Autodesk Inventor part; units mm, degrees
ref_plane "YZ Plane" through (0, 0, 0) normal (1, 0, 0) x (0, 1, 0)
ref_plane "XZ Plane" through (0, 0, 0) normal (0, 1, 0) x (-1, 0, 0)
ref_plane "XY Plane" through (0, 0, 0) normal (0, 0, 1) x (1, 0, 0)
sketch "スケッチ1" plane through (0, 0, 0) normal (1, 0, 0) x (0, 1, 0)
  line L0 (13.5, 13.5) -> (-13.5, 13.5)
  line L1 (-13.5, 13.5) -> (-13.5, -13.5)
  line L2 (-13.5, -13.5) -> (13.5, -13.5)
  line L3 (13.5, -13.5) -> (13.5, 13.5)
  circle A0 centre (0, 0) radius 6.5
  circle A1 centre (10.5, 10.5) radius 1.5
  circle A2 centre (10.5, -10.5) radius 1.5
  circle A3 centre (-10.5, -10.5) radius 1.5
  circle A4 centre (-10.5, 10.5) radius 1.5
  dimension "d0" = 27
  dimension "d1" = 27
  dimension "d2" = 13.5
  dimension "d3" = 13.5
  dimension "d4" = 13.5
  dimension "d5" = 13.5
  dimension "d6" = 13
  dimension "d7" = 3
  dimension "d8" = 3
  dimension "d9" = 3
  dimension "d10" = 3
  dimension "d11" = 3
  dimension "d12" = 3
  dimension "d13" = 3
  dimension "d14" = 3
  dimension "d15" = 3
  dimension "d16" = 3
  dimension "d17" = 3
  dimension "d18" = 3
extrude "押し出し1" add sketch "スケッチ1" along normal blind 2
extrude "押し出し2" add sketch "スケッチ1" along normal blind 25 contours A0
fillet "フィレット1" radius 6 1 edges at (25, -6.5, 0)
sketch "スケッチ2" plane through (2, 0, 0) normal (1, 0, 0) x (0, 0, -1)
  circle A0 centre (0, 10) radius 1.5
  circle A1 centre (-10, -6.5) radius 1.5
  circle A2 centre (10, -6.5) radius 1.3994
  line L0 (0, 10) -> (10, -6.5)
  line L1 (10, -6.5) -> (-10, -6.5)
  line L2 (0, 10) -> (-10, -6.5)
  line L3 (13.5, 13.5) -> (-13.5, 13.5)
  line L4 (13.5, -13.5) -> (13.5, 13.5)
  line L5 (-13.5, 13.5) -> (-13.5, -13.5)
  line L6 (-13.5, -13.5) -> (13.5, -13.5)
  point P0 (0, 0)
  dimension "d25" = 3.5
  dimension "d26" = 3.5
  dimension "d27" = 3.5
  dimension "d28" = 2.7988
  dimension "d29" = 7
  dimension "d30" = 3
  dimension "d31" = 3
extrude "押し出し3" add sketch "スケッチ2" along normal blind 16 contours A0 L0 L2 | L2 L0 A0 | A0 L0 A2 L1 A1 L2 | L2 L1 A1 | A1 L1 L2 | L0 L1 A2 | A2 L1 L0
properties part number "キャスター" material "PAEK 樹脂"
Here's how the part is built. I have some questions about the finished solid (model axes, mm). A direction names the side the tool comes from. Round coordinates to 2 decimals unless told otherwise and drop trailing zeros. Write each loop counter-clockwise with the first axis right and the second up, starting at its lowest first coordinate (ties: lowest second). Pieces come first, ordered by that corner, then holes.
Q1. If we section it at A-A on y = 10.5: Write out the boundary of the cut face in (x, z).
Q2. If we section it at D-D on y = 7: Write out the boundary of the cut face in (x, z).
Q3. If we mould it in two halves opening along Y, with no side actions, what happens to faces 1 (the cylindrical face through (1, 9.3, 11.4)), 2 (the flat face through (1, 13.5, 0)), 3 (the flat face through (25, 0, 0)), 4 (the flat face through (10, -6.5, 0))? For each: +Y half, -Y half, draft (parallel to the pull), parting line (faces both ways), or undercut.
Q4. If we section it at C-C on x = 10.5: Write out the boundary of the cut face in (y, z), plus the area to 3 significant figures.
Q5. Will these pins go through, and if not, where does the flat tip stop? P1, Ø3.5, axis at y = 10.5, z = 10.5, coming from the +X side; P2, Ø4, axis at y = 8, z = 0.5, coming from the +X side; P3, Ø6, axis at x = 6, y = -8, coming from the +Z side.
Q6. Which directions (+Z, -Z, +X, -X, +Y, -Y) give clear straight access to the entire face, cutting with the end or side of a thin tool? Please do faces 5 (the flat face through (9.888, 7.398, -1.577)), 6 (the flat face through (18, -5, 7)), 7 (the flat face through (2, 6, 3)), 8 (the flat face through (18, -5, -7)).
Q7. Please list where these lines run through material, in increasing order: probe 1 along Z at (x, y) = (0.5, 10.5); probe 2 along X at (y, z) = (6.25, 9.75); probe 3 along Y at (x, z) = (14.75, 1).
Q8. If we section it at B-B on z = -10: Write out the boundary of the cut face in (x, y), plus the area to 3 significant figures.
Answer below:
1. outline: (0, -13.5) - (2, -13.5) - (2, -12) - (0, -12) - close; (0, -9) - (2, -9) - (2, -1.41) - (18, -1.41) - (18, 1.41) - (2, 1.41) - (2, 9) - (0, 9) - close; (0, 12) - (2, 12) - (2, 13.5) - (0, 13.5) - close
2. outline: (0, -13.5) - (2, -13.5) - (2, -1.82) - (18, -1.82) - (18, 1.82) - (2, 1.82) - (2, 13.5) - (0, 13.5) - close
3. face 1: undercut
3. face 2: +Y half
3. face 3: draft
3. face 4: -Y half
4. outline: (-6.5, -8.6) arc R1.4 ccw (long way) to (-5.3, -9.27) - (-0.67, -6.47) arc R6.5 ccw to (6.04, -2.4) - (8.72, -0.78) arc R1.5 ccw (long way) to (8.72, 0.78) - (6.04, 2.4) arc R6.5 ccw to (-0.67, 6.47) - (-5.22, 9.22) arc R1.5 ccw (long way) to (-6.5, 8.5) - close
4. area: 196 mm2
5. P1: stops at x = 2
5. P2: stops at x = 21.36
5. P3: stops at z = 11.5
6. face 5: -Z, +X
6. face 6: +Z, +X, -Y
6. face 7: +X
6. face 8: -Z, +X, -Y
7. probe 1: z = -13.5 to -12, -9 to 9, 12 to 13.5
7. probe 2: x = 0 to 2
7. probe 3: y = -6.5 to 8.35, 8.88 to 11.12
8. outline: (0, -13.5) - (2, -13.5) - (2, -11.91) - (0, -11.91) - close; (0, -9.09) - (2, -9.09) - (2, -7.9) - (18, -7.9) - (18, -5.1) - (2, -5.1) - (2, 9.09) - (0, 9.09) - close; (0, 11.91) - (2, 11.91) - (2, 13.5) - (0, 13.5) - close
8. area: 87.5 mm2
